```python
from build123d import *

# Parameters (mm, degrees)
BOSS_EXTRUDE1_DEPTH = 60
SKETCH2_W           = 80
SKETCH2_H           = 65
CUT_EXTRUDE1_DEPTH  = 60
CUT_EXTRUDE2_REACH  = 142
SKETCH3_R           = 1.5
SKETCH3_R_2         = 5
CUT_EXTRUDE3_REACH  = 92
SKETCH4_R           = 5
SKETCH4_R_2         = 10
SKETCH4_R_3         = 2
FILLET1_R           = 2.5
FILLET3_R           = 2.5
FILLET4_R           = 2.5
FILLET5_R           = 2.5
FILLET6_R           = 2.5
SKETCH5_R           = 5
SKETCH5_R_2         = 2
CUT_EXTRUDE4_DEPTH  = 91
CUT_EXTRUDE5_REACH  = 92
SKETCH6_W           = 30
SKETCH6_H           = 10


with BuildPart() as part:
    # Sketch1 → Boss-Extrude1 (new body)
    with BuildSketch(Plane(origin=(0, 0, 0), x_dir=(0, 0, -1), z_dir=(1, 0, 0))):
        Polygon((0, 0), (0, -140), (-5, -140), (-5, -75), (-85, -75), (-85, -140), (-90, -140), (-90, 0), align=None)
    extrude(amount=-BOSS_EXTRUDE1_DEPTH)

    # Sketch2 → Cut-Extrude1 (cut)
    with BuildSketch(Plane(origin=(0, 0, 0), x_dir=(0, 0, -1), z_dir=(1, 0, 0))):
        with Locations((-45, -37.5)):
            Rectangle(SKETCH2_W, SKETCH2_H)
    extrude(amount=-CUT_EXTRUDE1_DEPTH, mode=Mode.SUBTRACT)

    # Sketch3 → Cut-Extrude2 (cut, up to next)
    with BuildSketch(Plane(origin=(0, 0, 0), x_dir=(1, 0, 0), z_dir=(0, 1, 0)), mode=Mode.PRIVATE) as cut_extrude2_sk1:
        with Locations((-35.5, -37)):
            Circle(SKETCH3_R)
    cut_extrude2_tool1 = extrude(cut_extrude2_sk1.sketch, amount=-CUT_EXTRUDE2_REACH, mode=Mode.PRIVATE) & part.part
    add(cut_extrude2_tool1.solids().sort_by_distance((-35.5, 0, 37))[0], mode=Mode.SUBTRACT)
    # Sketch3 → Cut-Extrude2 (cut, up to next)
    with BuildSketch(Plane(origin=(0, 0, 0), x_dir=(1, 0, 0), z_dir=(0, 1, 0)), mode=Mode.PRIVATE) as cut_extrude2_sk2:
        with Locations((-24.5, -37)):
            Circle(SKETCH3_R)
    cut_extrude2_tool2 = extrude(cut_extrude2_sk2.sketch, amount=-CUT_EXTRUDE2_REACH, mode=Mode.PRIVATE) & part.part
    add(cut_extrude2_tool2.solids().sort_by_distance((-24.5, 0, 37))[0], mode=Mode.SUBTRACT)
    # Sketch3 → Cut-Extrude2 (cut, up to next)
    with BuildSketch(Plane(origin=(0, 0, 0), x_dir=(1, 0, 0), z_dir=(0, 1, 0)), mode=Mode.PRIVATE) as cut_extrude2_sk3:
        with Locations((-24.5, -48)):
            Circle(SKETCH3_R)
    cut_extrude2_tool3 = extrude(cut_extrude2_sk3.sketch, amount=-CUT_EXTRUDE2_REACH, mode=Mode.PRIVATE) & part.part
    add(cut_extrude2_tool3.solids().sort_by_distance((-24.5, 0, 48))[0], mode=Mode.SUBTRACT)
    # Sketch3 → Cut-Extrude2 (cut, up to next)
    with BuildSketch(Plane(origin=(0, 0, 0), x_dir=(1, 0, 0), z_dir=(0, 1, 0)), mode=Mode.PRIVATE) as cut_extrude2_sk4:
        with Locations((-35.5, -48)):
            Circle(SKETCH3_R)
    cut_extrude2_tool4 = extrude(cut_extrude2_sk4.sketch, amount=-CUT_EXTRUDE2_REACH, mode=Mode.PRIVATE) & part.part
    add(cut_extrude2_tool4.solids().sort_by_distance((-35.5, 0, 48))[0], mode=Mode.SUBTRACT)
    # Sketch3 → Cut-Extrude2 (cut, up to next)
    with BuildSketch(Plane(origin=(0, 0, 0), x_dir=(1, 0, 0), z_dir=(0, 1, 0)), mode=Mode.PRIVATE) as cut_extrude2_sk5:
        with Locations((-30, -13)):
            Circle(SKETCH3_R_2)
    cut_extrude2_tool5 = extrude(cut_extrude2_sk5.sketch, amount=-CUT_EXTRUDE2_REACH, mode=Mode.PRIVATE) & part.part
    add(cut_extrude2_tool5.solids().sort_by_distance((-30, 0, 13))[0], mode=Mode.SUBTRACT)
    # Sketch3 → Cut-Extrude2 (cut, up to next)
    with BuildSketch(Plane(origin=(0, 0, 0), x_dir=(1, 0, 0), z_dir=(0, 1, 0)), mode=Mode.PRIVATE) as cut_extrude2_sk6:
        with Locations((-12, -32)):
            Circle(SKETCH3_R)
    cut_extrude2_tool6 = extrude(cut_extrude2_sk6.sketch, amount=-CUT_EXTRUDE2_REACH, mode=Mode.PRIVATE) & part.part
    add(cut_extrude2_tool6.solids().sort_by_distance((-12, 0, 32))[0], mode=Mode.SUBTRACT)
    # Sketch3 → Cut-Extrude2 (cut, up to next)
    with BuildSketch(Plane(origin=(0, 0, 0), x_dir=(1, 0, 0), z_dir=(0, 1, 0)), mode=Mode.PRIVATE) as cut_extrude2_sk7:
        with Locations((-48, -32)):
            Circle(SKETCH3_R)
    cut_extrude2_tool7 = extrude(cut_extrude2_sk7.sketch, amount=-CUT_EXTRUDE2_REACH, mode=Mode.PRIVATE) & part.part
    add(cut_extrude2_tool7.solids().sort_by_distance((-48, 0, 32))[0], mode=Mode.SUBTRACT)

    # Sketch4 → Cut-Extrude3 (cut, up to next)
    with BuildSketch(Plane.XY, mode=Mode.PRIVATE) as cut_extrude3_sk1:
        with Locations((-30, -112)):
            Circle(SKETCH4_R)
    cut_extrude3_tool1 = extrude(cut_extrude3_sk1.sketch, amount=CUT_EXTRUDE3_REACH, mode=Mode.PRIVATE) & part.part
    add(cut_extrude3_tool1.solids().sort_by_distance((-30, -112, 0))[0], mode=Mode.SUBTRACT)
    # Sketch4 → Cut-Extrude3 (cut, up to next)
    with BuildSketch(Plane.XY, mode=Mode.PRIVATE) as cut_extrude3_sk2:
        with Locations((-30, -40)):
            Circle(SKETCH4_R_2)
    cut_extrude3_tool2 = extrude(cut_extrude3_sk2.sketch, amount=CUT_EXTRUDE3_REACH, mode=Mode.PRIVATE) & part.part
    add(cut_extrude3_tool2.solids().sort_by_distance((-30, -40, 0))[0], mode=Mode.SUBTRACT)
    # Sketch4 → Cut-Extrude3 (cut, up to next)
    with BuildSketch(Plane.XY, mode=Mode.PRIVATE) as cut_extrude3_sk3:
        with Locations((-5, -82)):
            Circle(SKETCH4_R_3)
    cut_extrude3_tool3 = extrude(cut_extrude3_sk3.sketch, amount=CUT_EXTRUDE3_REACH, mode=Mode.PRIVATE) & part.part
    add(cut_extrude3_tool3.solids().sort_by_distance((-5, -82, 0))[0], mode=Mode.SUBTRACT)
    # Sketch4 → Cut-Extrude3 (cut, up to next)
    with BuildSketch(Plane.XY, mode=Mode.PRIVATE) as cut_extrude3_sk4:
        with Locations((-55, -82)):
            Circle(SKETCH4_R_3)
    cut_extrude3_tool4 = extrude(cut_extrude3_sk4.sketch, amount=CUT_EXTRUDE3_REACH, mode=Mode.PRIVATE) & part.part
    add(cut_extrude3_tool4.solids().sort_by_distance((-55, -82, 0))[0], mode=Mode.SUBTRACT)
    # Sketch4 → Cut-Extrude3 (cut, up to next)
    with BuildSketch(Plane.XY, mode=Mode.PRIVATE) as cut_extrude3_sk5:
        with Locations((-14.5, -24.5)):
            Circle(SKETCH4_R_3)
    cut_extrude3_tool5 = extrude(cut_extrude3_sk5.sketch, amount=CUT_EXTRUDE3_REACH, mode=Mode.PRIVATE) & part.part
    add(cut_extrude3_tool5.solids().sort_by_distance((-14.5, -24.5, 0))[0], mode=Mode.SUBTRACT)
    # Sketch4 → Cut-Extrude3 (cut, up to next)
    with BuildSketch(Plane.XY, mode=Mode.PRIVATE) as cut_extrude3_sk6:
        with Locations((-45.5, -24.5)):
            Circle(SKETCH4_R_3)
    cut_extrude3_tool6 = extrude(cut_extrude3_sk6.sketch, amount=CUT_EXTRUDE3_REACH, mode=Mode.PRIVATE) & part.part
    add(cut_extrude3_tool6.solids().sort_by_distance((-45.5, -24.5, 0))[0], mode=Mode.SUBTRACT)
    # Sketch4 → Cut-Extrude3 (cut, up to next)
    with BuildSketch(Plane.XY, mode=Mode.PRIVATE) as cut_extrude3_sk7:
        with Locations((-45.5, -55.5)):
            Circle(SKETCH4_R_3)
    cut_extrude3_tool7 = extrude(cut_extrude3_sk7.sketch, amount=CUT_EXTRUDE3_REACH, mode=Mode.PRIVATE) & part.part
    add(cut_extrude3_tool7.solids().sort_by_distance((-45.5, -55.5, 0))[0], mode=Mode.SUBTRACT)
    # Sketch4 → Cut-Extrude3 (cut, up to next)
    with BuildSketch(Plane.XY, mode=Mode.PRIVATE) as cut_extrude3_sk8:
        with Locations((-14.5, -55.5)):
            Circle(SKETCH4_R_3)
    cut_extrude3_tool8 = extrude(cut_extrude3_sk8.sketch, amount=CUT_EXTRUDE3_REACH, mode=Mode.PRIVATE) & part.part
    add(cut_extrude3_tool8.solids().sort_by_distance((-14.5, -55.5, 0))[0], mode=Mode.SUBTRACT)

    # Fillet1
    fillet1_edges = [part.edges().sort_by_distance(p)[0] for p in [
        (-30, -75, 85),
    ]]
    fillet(fillet1_edges, radius=FILLET1_R)

    # Fillet3
    fillet3_edges = [part.edges().sort_by_distance(p)[0] for p in [
        (-30, -70, 85),
    ]]
    fillet(fillet3_edges, radius=FILLET3_R)

    # Fillet4
    fillet4_edges = [part.edges().sort_by_distance(p)[0] for p in [
        (-30, -70, 5),
    ]]
    fillet(fillet4_edges, radius=FILLET4_R)

    # Fillet5
    fillet5_edges = [part.edges().sort_by_distance(p)[0] for p in [
        (-30, -5, 5),
    ]]
    fillet(fillet5_edges, radius=FILLET5_R)

    # Fillet6
    fillet6_edges = [part.edges().sort_by_distance(p)[0] for p in [
        (-30, -5, 85),
    ]]
    fillet(fillet6_edges, radius=FILLET6_R)

    # Sketch5 → Cut-Extrude4 (cut, through all)
    with BuildSketch(Plane.XY.offset(90)):
        with Locations((-30, -112)):
            Circle(SKETCH5_R)
        with Locations((-12, -112)):
            Circle(SKETCH5_R_2)
        with Locations((-48, -112)):
            Circle(SKETCH5_R_2)
    extrude(amount=-CUT_EXTRUDE4_DEPTH, mode=Mode.SUBTRACT)

    # Sketch6 → Cut-Extrude5 (cut, up to next)
    with BuildSketch(Plane(origin=(0, 0, 0), x_dir=(-1, 0, 0), z_dir=(0, 0, -1)), mode=Mode.PRIVATE) as cut_extrude5_sk1:
        with Locations((15, -40)):
            Rectangle(SKETCH6_W, SKETCH6_H)
    cut_extrude5_tool1 = extrude(cut_extrude5_sk1.sketch, amount=-CUT_EXTRUDE5_REACH, mode=Mode.PRIVATE) & part.part
    add(cut_extrude5_tool1.solids().sort_by_distance((-15, -40, 0))[0], mode=Mode.SUBTRACT)


solid = part.part
```
Geometry: final body of the model. Coordinates: model frame, mm. A direction names the side the tool comes from. Round coordinates to 2 decimals unless told otherwise and drop trailing zeros. Order: outer loops, then holes, each group sorted by start corner. A loop starts at its lowest first (then second) coordinate and runs counter-clockwise, first axis right, second up. Notation, with made-up numbers: (63.25, -24) -> (99.25, -24) arc R13 cw to (99.25, -10) -> close; hole circle Ø8 at (64.25, 4). An arc over 180 degrees is marked (long way). Use CSV: the item, a comma, the result in double quotes. Start each with the question number.
1) Section A-A (y = -14). Return the cut outline in (x, z), and give its area (3 significant figures).
2) Set-up query: faces 5 (the face through (-43.653, -25.266, 2.465)), 6 (the face through (-23, -108, 5)), 7 (the face through (-11, -45, 2)), 8 (the face through (-35.825, -2.465, 49.464)), 9 (the face through (-30, -70, 46)). Return all of +Z, -Z, +X, -X, +Y, -Y with unobstructed straight access to the full face (end or side cutting, diameter ignored); none if empty.
3) Draft query along Y for faces 1 (the face through (-30, -140, 2)), 2 (the face through (-10.925, -110.314, 2.535)), 3 (the face through (-25.7, -2.5, 37.9)), 4 (the face through (-5, -80, 2)). Return one class per face: +Y half, -Y half, draft (parallel to the pull), parting line (faces both ways), or undercut.
4) Section B-B (z = 27.5). Return the cut outline in (x, y), and give its area (3 significant figures).
5) Material intervals for line 1 along X through (y, z) = (-3.2, 32); line 2 along Z through (x, y) = (-35.5, -2.7); line 3 along Y through (x, z) = (-14.5, 2.95), sorted ascending. Write a range as from..to.
6) Section D-D (x = -5). Return the cut outline in (y, z).
7) Section C-C (x = -51.5). Return the cut outline in (y, z).
8) First-contact query: pin 1 Ø12 at (x, y) = (-30, -40) entering from -Z; pin 2 Ø12 at (x, z) = (-46.5, 32.5) entering from -Y. Flat tips, straight axial feed; report the tip coordinate or a pass-through.
Returned:
1,outline,"(-60, 0) -> (0, 0) -> (0, 5) -> (-60, 5) -> close; (-60, 85) -> (0, 85) -> (0, 90) -> (-60, 90) -> close"
1,area,"600 mm²"
2,face 5,"-Z"
2,face 6,"+X, -X, -Y"
2,face 7,"-Z, +X"
2,face 8,"+Y"
2,face 9,"+X, -X"
3,face 1,"-Y half"
3,face 2,"undercut"
3,face 3,"draft"
3,face 4,"undercut"
4,outline,"(-60, -75) -> (0, -75) -> (0, -70) -> (-60, -70) -> close; (-60, -5) -> (0, -5) -> (0, 0) -> (-60, 0) -> close"
4,area,"600 mm²"
5,line 1,"x = -60..-49.5, -46.5..-13.5, -10.5..0"
5,line 2,"z = 0..35.5, 38.5..46.5, 49.5..90"
5,line 3,"y = -140..-57.5, -53.5..-45, -35..-26.5, -22.5..0"
6,outline,"(-140, 0) -> (-84, 0) -> (-84, 5) -> (-140, 5) -> close; (-140, 85) -> (-77.5, 85) arc R2.5 cw to (-75, 82.5) -> (-75, 5) -> (-80, 5) -> (-80, 0) -> (-45, 0) -> (-45, 5) -> (-67.5, 5) arc R2.5 cw to (-70, 7.5) -> (-70, 82.5) arc R2.5 cw to (-67.5, 85) -> (-7.5, 85) arc R2.5 cw to (-5, 82.5) -> (-5, 7.5) arc R2.5 cw to (-7.5, 5) -> (-35, 5) -> (-35, 0) -> (0, 0) -> (0, 90) -> (-140, 90) -> close"
7,outline,"(-140, 0) -> (0, 0) -> (0, 90) -> (-140, 90) -> (-140, 85) -> (-77.5, 85) arc R2.5 cw to (-75, 82.5) -> (-75, 5) -> (-140, 5) -> close; hole (-70, 7.5) arc R2.5 ccw to (-67.5, 5) -> (-7.5, 5) arc R2.5 ccw to (-5, 7.5) -> (-5, 82.5) arc R2.5 ccw to (-7.5, 85) -> (-67.5, 85) arc R2.5 ccw to (-70, 82.5) -> close"
8,pin 1,"stops at z = 85"
8,pin 2,"stops at y = -75"
